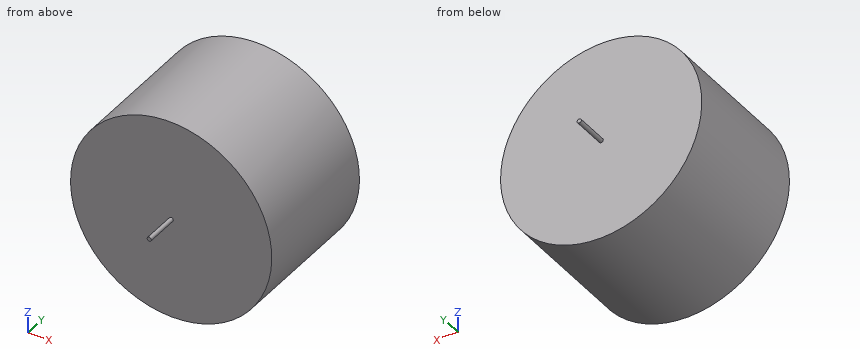
```python
from build123d import *

# Parameters (mm, degrees)
SKETCH1_R                = 457.2
BOSS_EXTRUDE1_DEPTH      = 609.6
BOSS_EXTRUDE2_DEPTH      = 152.4
BOSS_EXTRUDE2_DEPTH_BACK = 762
SKETCH2_R                = 9.525


with BuildPart() as part:
    # Sketch1 → Boss-Extrude1 (new body)
    with BuildSketch(Plane(origin=(0, 0, 0), x_dir=(1, 0, 0), z_dir=(0, 1, 0))):
        with Locations(Location((0, 0, 0), (0, 0, 90))):
            Circle(SKETCH1_R)
    extrude(amount=BOSS_EXTRUDE1_DEPTH)

    # Sketch2 → Boss-Extrude2 (add, two sides: drawn at the far end of the back side and taken through both)
    with BuildSketch(Plane(origin=(0, 609.6, 0), x_dir=(1, 0, 0), z_dir=(0, 1, 0)).offset(-BOSS_EXTRUDE2_DEPTH_BACK)):
        with Locations(Location((0, 0, 0), (0, 0, 270))):
            Circle(SKETCH2_R)
    extrude(amount=BOSS_EXTRUDE2_DEPTH + BOSS_EXTRUDE2_DEPTH_BACK)


solid = part.part
```
Can you work these out from the model? Positions are in its coordinate system, mm. Coordinates: 2 decimals unless noted, no trailing zeros. Loops run counter-clockwise (first coordinate to the right, second up) from the corner with the lowest first, then second, coordinate; pieces in that order, holes last. Notation, with made-up numbers: M 89.25,82.25 L 141.25,82.25 A15 ccw 141.25,100.25 Z; hole C 74,-16 d9. An arc over 180 degrees is marked long. Put each result on its own line as item: value. Start each with the question number.
(1) Will these pins go through, and if not, where does the flat tip stop? pin 1 Ø6 at (x, y) = (-126.5, 15.5) entering from -Z; pin 2 Ø4 at (x, y) = (-336, 204.5) entering from -Z; pin 3 Ø1 at (x, z) = (-24.5, 162) entering from +Y.
(2) I need wall thicknesses on probe 1 along Y at (x, z) = (-162, -94.5); probe 2 along X at (y, z) = (501, -137); probe 3 along X at (y, z) = (55, -126). Which ranges of each line are inside material? Lowest first, please.
(3) Imagine slicing it at C-C on z = 162. List the corners of the cut face in (x, y) for me, and give its area (3 significant figures).
(4) Imagine slicing it at B-B on x = -316. List the corners of the cut face in (y, z) for me.
(5) Imagine slicing it at A-A on y = 88.5. List the corners of the cut face in (x, z) for me.
Worked answers:
1. pin 1: stops at z = -440.2
1. pin 2: stops at z = -312.21
1. pin 3: stops at y = 609.6
2. probe 1: y = 0 to 609.6
2. probe 2: x = -436.19 to 436.19
2. probe 3: x = -439.49 to 439.49
3. outline: M -427.54,0 L 427.54,0 L 427.54,609.6 L -427.54,609.6 Z
3. area: 521,000 mm2
4. outline: M 0,-330.42 L 609.6,-330.42 L 609.6,330.42 L 0,330.42 Z
5. outline: C 0,0 d914.4
